Verification items for the finished model (mm, model axes). A direction names the side the tool comes from. Coordinates: 2 decimals unless noted, no trailing zeros. Order: outer loops, then holes, each group sorted by start corner. A loop starts at its lowest first (then second) coordinate and runs counter-clockwise, first axis right, second up.
Q1. Thickness scan on line 1 (X direction, y = -2, z = 2.15); line 2 (X direction, y = -8.5, z = 0.7); line 3 (Y direction, x = -16.5, z = 1.2). Record the ranges inside material, lowest first.
Q2. Set-up check for faces 1 (the flat face through (22, -12, 1)), 2 (the flat face through (-10, 12, 1)): record each of +Z, -Z, +X, -X, +Y, -Y from which the full face is reachable in a straight line by a thin tool's end or side.
Q3. Cross-section at A-A, the plane x = -20. Record the boundary of the cut face in (y, z), and give its area (3 significant figures).
Q4. Draft check along Y on faces 3 (the flat face through (-5.7, 0.2, 0)), 4 (the flat face through (-21, -13, 1)), 5 (the flat face through (-19, 5, 1)). Enter one of: pulls with the +Y half, pulls with the -Y half, needs draft (parallel to the pull), parting line crosses it, or undercut.
Q5. Cross-section at C-C, the plane z = 2.05. Record the boundary of the cut face in (x, y), and give its area (3 significant figures).
Q6. Cross-section at B-B, the plane y = 10.5. Record the boundary of the cut face in (x, z), and give its area (3 significant figures).
Q7. Cross-section at D-D, the plane y = 2. Record the boundary of the cut face in (x, z).
from build123d import *

# Parameters (mm, degrees)
F0_W     = 7
F0_H     = 24
F0_W_2   = 48
F0_H_2   = 30
F0_H_3   = 10
F1_DEPTH = 2.5
F2_DEPTH = 2.5
F3_SIZE2 = 5
F3_SIZE  = 5


with BuildPart() as f1:
    # F0 (on Top) → F1 (new body)
    with BuildSketch(Plane.XY):
        with Locations((9.5, 0)):
            Rectangle(F0_W, F0_H)
        Rectangle(F0_W_2, F0_H_2)
        with Locations((-18.5, 0)):
            Rectangle(F0_W, F0_H_3, mode=Mode.SUBTRACT)
        with Locations((-9.5, 0)):
            Rectangle(F0_W, F0_H, mode=Mode.SUBTRACT)
        Rectangle(F0_W, F0_H, mode=Mode.SUBTRACT)
        with Locations((9.5, 0)):
            Rectangle(F0_W, F0_H, mode=Mode.SUBTRACT)
        with Locations((18.5, 0)):
            Rectangle(F0_W, F0_H_3, mode=Mode.SUBTRACT)
        with Locations((-18.5, 0)):
            Rectangle(F0_W, F0_H_3)
        with Locations((-9.5, 0)):
            Rectangle(F0_W, F0_H)
        Rectangle(F0_W, F0_H)
        with Locations((18.5, 0)):
            Rectangle(F0_W, F0_H_3)
    extrude(amount=F1_DEPTH)

    # F0 (on Top) → F2 (cut)
    with BuildSketch(Plane.XY):
        with Locations((-18.5, 0)):
            Rectangle(F0_W, F0_H_3)
        with Locations((18.5, 0)):
            Rectangle(F0_W, F0_H_3)
        with Locations((-9.5, 0)):
            Rectangle(F0_W, F0_H)
        Rectangle(F0_W, F0_H)
        with Locations((9.5, 0)):
            Rectangle(F0_W, F0_H)
    extrude(amount=F2_DEPTH, mode=Mode.SUBTRACT)

    # F3
    f3_edges = [f1.edges().sort_by_distance(p)[0] for p in [
        (24, -15, 1.25),
        (24, 15, 1.25),
        (-24, 15, 1.25),
        (-24, -15, 1.25),
    ]]
    chamfer(f3_edges, length=F3_SIZE, length2=F3_SIZE2)


solid = f1.part
Check values:
1. line 1: x = -24 to -22, -15 to -13, -6 to -3.5, 3.5 to 6, 13 to 15, 22 to 24
1. line 2: x = -24 to -13, -6 to -3.5, 3.5 to 6, 13 to 24
1. line 3: y = -15 to -5, 5 to 15
2. face 1: +Z, -Z, +X, -Y
2. face 2: +Z, -Z
3. outline: (-14, 0) - (-5, 0) - (-5, 2.5) - (-14, 2.5) - close; (5, 0) - (14, 0) - (14, 2.5) - (5, 2.5) - close
3. area: 45.0 mm2
4. face 3: needs draft
4. face 4: pulls with the -Y half
4. face 5: undercut
5. outline: (-24, -10) - (-19, -15) - (19, -15) - (24, -10) - (24, 10) - (19, 15) - (-19, 15) - (-24, 10) - close; hole (-22, -5) - (-15, -5) - (-15, 5) - (-22, 5) - close; hole (-13, -12) - (-6, -12) - (-6, 12) - (-13, 12) - close; hole (-3.5, -12) - (3.5, -12) - (3.5, 12) - (-3.5, 12) - close; hole (6, -12) - (13, -12) - (13, 12) - (6, 12) - close; hole (15, -5) - (22, -5) - (22, 5) - (15, 5) - close
5. area: 746 mm2
6. outline: (-23.5, 0) - (-13, 0) - (-13, 2.5) - (-23.5, 2.5) - close; (-6, 0) - (-3.5, 0) - (-3.5, 2.5) - (-6, 2.5) - close; (3.5, 0) - (6, 0) - (6, 2.5) - (3.5, 2.5) - close; (13, 0) - (23.5, 0) - (23.5, 2.5) - (13, 2.5) - close
6. area: 65.0 mm2
7. outline: (-24, 0) - (-22, 0) - (-22, 2.5) - (-24, 2.5) - close; (-15, 0) - (-13, 0) - (-13, 2.5) - (-15, 2.5) - close; (-6, 0) - (-3.5, 0) - (-3.5, 2.5) - (-6, 2.5) - close; (3.5, 0) - (6, 0) - (6, 2.5) - (3.5, 2.5) - close; (13, 0) - (15, 0) - (15, 2.5) - (13, 2.5) - close; (22, 0) - (24, 0) - (24, 2.5) - (22, 2.5) - close
